```python
from build123d import *

# Parameters (mm, degrees)
SKETCH1_R           = 2.1
BOSS_EXTRUDE1_DEPTH = 6
SKETCH2_R           = 2.1
BOSS_EXTRUDE2_DEPTH = 9
SKETCH3_W           = 5
SKETCH3_H           = 28
CUT_EXTRUDE1_DEPTH  = 38.536648758


with BuildPart() as part:
    # Sketch1 → Boss-Extrude1 (new body)
    with BuildSketch(Plane(origin=(0, 0, 0), x_dir=(1, 0, 0), z_dir=(0, 1, 0))):
        with BuildLine():
            Line((22.603957871, 7.564350825), (1.952968403, 14.673263119))
            ThreePointArc((1.952968403, 14.673263119), (0.990055879, 14.917752053), (0, 15))
            Line((0, 15), (0, -15))
            ThreePointArc((0, -15), (2.077420969, -14.818812213), (4.092108053, -14.280720353))
            Line((4.092108053, -14.280720353), (22.728072035, -7.520480235))
            ThreePointArc((22.728072035, -7.520480235), (27.999729231, 0.065819743), (22.603957871, 7.564350825))
        make_face()
        with Locations(Location((20, 0, 0), (0, 0, 270))):
            Circle(SKETCH1_R, mode=Mode.SUBTRACT)
    boss_extrude1 = extrude(amount=BOSS_EXTRUDE1_DEPTH)

    # Mirror1: Boss-Extrude1 across plane
    add(boss_extrude1.mirror(Plane(origin=(0, 6, -15), x_dir=(0, 0, 1), z_dir=(1, 0, 0))))

    # Sketch2 → Boss-Extrude2 (add, symmetric)
    with BuildSketch(Plane(origin=(0, 0, 0), x_dir=(0, 0, -1), z_dir=(1, 0, 0))):
        with BuildLine():
            Line((-6, 6), (-3.92777975, 16.75666785))
            ThreePointArc((-3.92777975, 16.75666785), (0, 20), (3.92777975, 16.75666785))
            Line((3.92777975, 16.75666785), (6, 6))
            Line((6, 6), (-6, 6))
        make_face()
        with Locations((0, 16)):
            Circle(SKETCH2_R, mode=Mode.SUBTRACT)
    extrude(amount=BOSS_EXTRUDE2_DEPTH, both=True)

    # Sketch3 → Cut-Extrude1 (cut, symmetric)
    with BuildSketch(Plane.XY):
        with Locations((-5, 20)):
            Rectangle(SKETCH3_W, SKETCH3_H)
    cut_extrude1 = extrude(amount=CUT_EXTRUDE1_DEPTH, both=True, mode=Mode.SUBTRACT)

    # Mirror2: Cut-Extrude1 across plane
    add(cut_extrude1.mirror(Plane(origin=(0, 0, 0), x_dir=(0, 0, 1), z_dir=(1, 0, 0))), mode=Mode.SUBTRACT)


solid = part.part
```
Here's how the part is built. I have some questions about the finished solid (model axes, mm). A direction names the side the tool comes from. Coordinates: 2 decimals unless noted, no trailing zeros. Write each loop counter-clockwise with the first axis right and the second up, starting at its lowest first coordinate (ties: lowest second). Pieces come first, ordered by that corner, then holes. Notation, with made-up numbers: (67, -16.75) -> (112, -16.75) arc R11 cw to (112, -2.75) -> close; hole circle Ø6 at (38, -37.75). An arc over 180 degrees is marked (long way). Use a Markdown table: item, result. Add a question column.
(1) I'm going to push flat-ended pins straight in: P1, Ø6, axis at x = -17.5, z = -11.5, coming from the +Y side; P2, Ø5.5, axis at y = 16, z = 0, coming from the +X side; P3, Ø6, axis at y = 12, z = -1, coming from the -X side; P4, Ø12, axis at x = 4, z = -4.5, coming from the -Y side. Where does each tip first touch, or does it pass through?
(2) If we section it at C-C, the plane y = 4: Write out the boundary of the cut face in (x, z), and give its area (3 significant figures).
(3) Please list where these lines run through material, in increasing order: line 1 (X direction, y = 19, z = 0.75); line 2 (X direction, y = 4.7, z = 0); line 3 (Y direction, x = -0.45, z = 0).
(4) For faces 1 (the flat face through (9, 12, 0)), 2 (the flat face through (7.5, 11, 0)), 3 (the flat face through (-9, 12, 0)), which set-ups out of +Z, -Z, +X, -X, +Y, -Y let a thin tool reach every point of the face, with its end or its side?
(5) If we section it at B-B, the plane x = -20: Write out the boundary of the cut face in (y, z).
(6) We'd pull the mould along Z, two halves only. Please class faces 4 (the flat face through (0, 0, 0)), 5 (the cylindrical face through (-0.04, 17.77, -1.13)), 6 (the cylindrical face through (-28, 3, 0)): +Z half, -Z half, draft (parallel to the pull), parting line (faces both ways), or undercut.
(7) If we section it at A-A, the plane y = 15: Write out the boundary of the cut face in (x, z).
(8) If we section it at D-D, the plane z = 0: State how many separate pieces and enclosed holes the cut face has, and give its area (3 significant figures).
Outcome:
| question | item | result |
|---|---|---|
| 1 | P1 | stops at y = 6 |
| 1 | P2 | stops at x = 9 |
| 1 | P3 | stops at x = -9 |
| 1 | P4 | stops at y = 0 |
| 2 | outline | (-22.73, 7.52) arc R8 ccw to (-22.6, -7.56) -> (-1.95, -14.67) arc R6 ccw to (1.95, -14.67) -> (22.6, -7.56) arc R8 ccw to (22.73, 7.52) -> (4.09, 14.28) arc R12 ccw to (-4.09, 14.28) -> close; hole circle Ø4.2 at (-20, 0); hole circle Ø4.2 at (20, 0) |
| 2 | area | 1,130 mm^2 |
| 3 | line 1 | x = -9 to -7.5, -2.5 to 2.5, 7.5 to 9 |
| 3 | line 2 | x = -28 to -22.1, -17.9 to 17.9, 22.1 to 28 |
| 3 | line 3 | y = 0 to 13.9, 18.1 to 20 |
| 4 | face 1 | +Z, -Z, +X, +Y |
| 4 | face 2 | +Z, -Z, +Y |
| 4 | face 3 | +Z, -Z, -X, +Y |
| 5 | outline | (0, -8.46) -> (6, -8.46) -> (6, -2.1) -> (0, -2.1) -> close; (0, 2.1) -> (6, 2.1) -> (6, 8.51) -> (0, 8.51) -> close |
| 6 | face 4 | draft |
| 6 | face 5 | undercut |
| 6 | face 6 | parting line |
| 7 | outline | (-9, -4.27) -> (-7.5, -4.27) -> (-7.5, -1.85) -> (-9, -1.85) -> close; (-9, 1.85) -> (-7.5, 1.85) -> (-7.5, 4.27) -> (-9, 4.27) -> close; (-2.5, -4.27) -> (2.5, -4.27) -> (2.5, -1.85) -> (-2.5, -1.85) -> close; (-2.5, 1.85) -> (2.5, 1.85) -> (2.5, 4.27) -> (-2.5, 4.27) -> close; (7.5, -4.27) -> (9, -4.27) -> (9, -1.85) -> (7.5, -1.85) -> close; (7.5, 1.85) -> (9, 1.85) -> (9, 4.27) -> (7.5, 4.27) -> close |
| 8 | separate pieces | 6 |
| 8 | enclosed holes | 0 |
| 8 | area | 364 mm^2 |
